Part model, mm, in its own coordinate system. Face numbers are marked on the shaded views. A direction names the side the tool comes from. Coordinates: 2 decimals unless noted, no trailing zeros. Write each loop counter-clockwise with the first axis right and the second up, starting at its lowest first coordinate (ties: lowest second). Pieces come first, ordered by that corner, then holes. Notation, with made-up numbers: (15, 63.25) - (36, 63.25) arc R17 cw to (36, 88.25) - close; hole circle Ø9 at (-33, -0.5). An arc over 180 degrees is marked (long way). Use a Markdown table: item, result.
```python
from build123d import *

# Parameters (mm, degrees)
SKETCH1_W                = 40
SKETCH1_H                = 20
SKETCH1_R                = 4
SKETCH1_H_2              = 10
SKETCH1_W_2              = 20
SKETCH1_H_3              = 4.76
BOSS_EXTRUDE1_DEPTH      = 3
SKETCH1_5_W              = 40
SKETCH1_5_H              = 20
SKETCH1_5_R              = 4
SKETCH1_5_H_2            = 10
SKETCH1_5_W_2            = 20
SKETCH1_5_H_3            = 4.76
BOSS_EXTRUDE3_DEPTH      = 7.5
SKETCH1_6_W              = 40
SKETCH1_6_H              = 20
SKETCH1_6_R              = 4
CUT_EXTRUDE1_DEPTH       = 4.5
SKETCH1_7_W              = 40
SKETCH1_7_H              = 10
SKETCH1_7_W_2            = 20
SKETCH1_7_H_2            = 4.76
BOSS_EXTRUDE4_DEPTH      = 18
BOSS_EXTRUDE4_DEPTH_BACK = 20.5
SKETCH5_R                = 4
CUT_EXTRUDE2_DEPTH       = 10


with BuildPart() as part:
    # Sketch1 → Boss-Extrude1 (new body)
    with BuildSketch(Plane.XY):
        with Locations((-26.342010442, -110)):
            Rectangle(SKETCH1_W, SKETCH1_H)
        with Locations((-36.342010442, -110)):
            Circle(SKETCH1_R, mode=Mode.SUBTRACT)
        with Locations((-16.342010442, -110)):
            Circle(SKETCH1_R, mode=Mode.SUBTRACT)
        with Locations((-26.342010442, -125)):
            Rectangle(SKETCH1_W, SKETCH1_H_2)
        with Locations((-26.342010442, -125)):
            Rectangle(SKETCH1_W_2, SKETCH1_H_3, mode=Mode.SUBTRACT)
    extrude(amount=BOSS_EXTRUDE1_DEPTH)

    # Sketch1_5 → Boss-Extrude3 (add)
    with BuildSketch(Plane.XY):
        with Locations((-26.342010442, -110)):
            Rectangle(SKETCH1_5_W, SKETCH1_5_H)
        with Locations((-36.342010442, -110)):
            Circle(SKETCH1_5_R, mode=Mode.SUBTRACT)
        with Locations((-16.342010442, -110)):
            Circle(SKETCH1_5_R, mode=Mode.SUBTRACT)
        with Locations((-26.342010442, -125)):
            Rectangle(SKETCH1_5_W, SKETCH1_5_H_2)
        with Locations((-26.342010442, -125)):
            Rectangle(SKETCH1_5_W_2, SKETCH1_5_H_3, mode=Mode.SUBTRACT)
    extrude(amount=-BOSS_EXTRUDE3_DEPTH)

    # Sketch1_6 → Cut-Extrude1 (cut)
    with BuildSketch(Plane.XY):
        with Locations((-26.342010442, -110)):
            Rectangle(SKETCH1_6_W, SKETCH1_6_H)
        with Locations((-36.342010442, -110)):
            Circle(SKETCH1_6_R, mode=Mode.SUBTRACT)
        with Locations((-16.342010442, -110)):
            Circle(SKETCH1_6_R, mode=Mode.SUBTRACT)
    extrude(amount=-CUT_EXTRUDE1_DEPTH, mode=Mode.SUBTRACT)

    # Sketch1_7 → Boss-Extrude4 (add, two sides)
    with BuildSketch(Plane.XY) as boss_extrude4_sk:
        with Locations((-26.342010442, -125)):
            Rectangle(SKETCH1_7_W, SKETCH1_7_H)
        with Locations((-26.342010442, -125)):
            Rectangle(SKETCH1_7_W_2, SKETCH1_7_H_2, mode=Mode.SUBTRACT)
    extrude(amount=BOSS_EXTRUDE4_DEPTH)
    extrude(boss_extrude4_sk.sketch, amount=-BOSS_EXTRUDE4_DEPTH_BACK)

    # Sketch5 → Cut-Extrude2 (cut)
    with BuildSketch(Plane.XZ.offset(130)):
        with Locations((-26.342010442, 11)):
            Circle(SKETCH5_R)
        with Locations((-26.342010442, -13.5)):
            Circle(SKETCH5_R)
    extrude(amount=-CUT_EXTRUDE2_DEPTH, mode=Mode.SUBTRACT)


solid = part.part
```
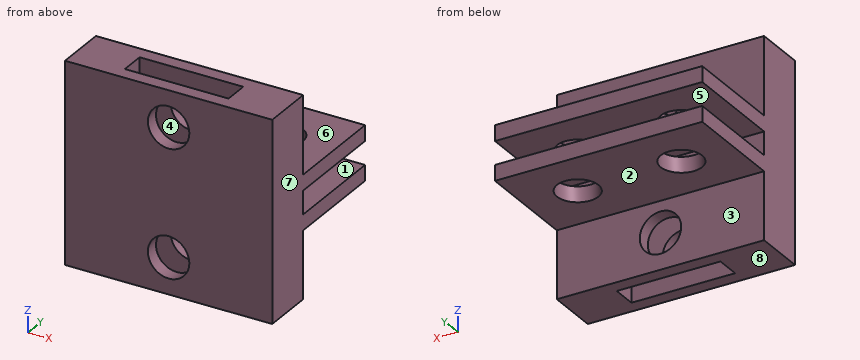
Item 1: Band-saw the part on C-C, the plane y = -110. Give the cut face in (x, z).
From the geometry:
| item | result |
|---|---|
| outline | (-46.34, -7.5) - (-40.34, -7.5) - (-40.34, -4.5) - (-46.34, -4.5) - close; (-46.34, 0) - (-40.34, 0) - (-40.34, 3) - (-46.34, 3) - close; (-32.34, -7.5) - (-20.34, -7.5) - (-20.34, -4.5) - (-32.34, -4.5) - close; (-32.34, 0) - (-20.34, 0) - (-20.34, 3) - (-32.34, 3) - close; (-12.34, -7.5) - (-6.34, -7.5) - (-6.34, -4.5) - (-12.34, -4.5) - close; (-12.34, 0) - (-6.34, 0) - (-6.34, 3) - (-12.34, 3) - close |
Item 2: Two-plate mould, pull along Z, no slides. Class the marked faces 1, 2 and 3: pulls with the +Z half, pulls with the -Z half, needs draft (parallel to the pull), parting line crosses it, or undercut.
From the geometry:
| item | result |
|---|---|
| face 1 | undercut |
| face 2 | pulls with the -Z half |
| face 3 | needs draft |
Item 3: Drop flat-ended pins along their axis: P1, Ø10.5, axis at x = -26.34, z = 11, coming from the -Y side; P2, Ø10, axis at x = -20, y = -110, coming from the -Z side; P3, Ø3.5, axis at x = -21, z = -2, coming from the +Y side; P4, Ø1.5, axis at x = -37, y = -107.5, coming from the -Z side. Give the stop position or say it passes through.
From the geometry:
| item | result |
|---|---|
| P1 | y = -130 |
| P2 | z = -7.5 |
| P3 | y = -120 |
| P4 | through |
Item 4: Which spindle directions (+Z, -Z, +X, -X, +Y, -Y) get a long thin tool onto all of the face, cutting with end or side? Do the marked faces 4, 5, 6, 7 and 8. Say none if no direction does.
From the geometry:
| item | result |
|---|---|
| face 4 | +Z, -Z |
| face 5 | +X, -X, +Y |
| face 6 | +Z, +X, -X, +Y |
| face 7 | +Z, -Z, +X, +Y, -Y |
| face 8 | -Z, +X, -X, +Y, -Y |
Item 5: Band-saw the part on B-B, the plane z = 11. Give the cut face in (x, y), then the cut area to 3 significant figures.
From the geometry:
| item | result |
|---|---|
| outline | (-46.34, -130) - (-30.34, -130) - (-30.34, -127.38) - (-36.34, -127.38) - (-36.34, -122.62) - (-30.34, -122.62) - (-30.34, -120) - (-46.34, -120) - close; (-22.34, -130) - (-6.34, -130) - (-6.34, -120) - (-22.34, -120) - (-22.34, -122.62) - (-16.34, -122.62) - (-16.34, -127.38) - (-22.34, -127.38) - close |
| area | 263 mm^2 |
Item 6: Band-saw the part on A-A, the plane y = -102.75. Give the cut face in (x, z), then the cut area to 3 significant figures.
From the geometry:
| item | result |
|---|---|
| outline | (-46.34, -7.5) - (-6.34, -7.5) - (-6.34, -4.5) - (-46.34, -4.5) - close; (-46.34, 0) - (-6.34, 0) - (-6.34, 3) - (-46.34, 3) - close |
| area | 240 mm^2 |
Item 7: Band-saw the part on D-D, the plane x = -27. Count the separate pieces of the cut face and the enclosed holes in it, then the cut area to 3 significant figures.
From the geometry:
| item | result |
|---|---|
| separate pieces | 6 |
| enclosed holes | 0 |
| area | 239 mm^2 |
Item 8: Drill centre lines: probe 1 along Z at (x, y) = (-29.5, -121.75); probe 2 along X at (y, z) = (-124.5, -9); probe 3 along Z at (x, y) = (-18, -101.75). Where is each one in solid material? Low to high.
From the geometry:
| item | result |
|---|---|
| probe 1 | -20.5 to -15.96, -11.04 to 8.54, 13.46 to 18 |
| probe 2 | -46.34 to -36.34, -16.34 to -6.34 |
| probe 3 | -7.5 to -4.5, 0 to 3 |
